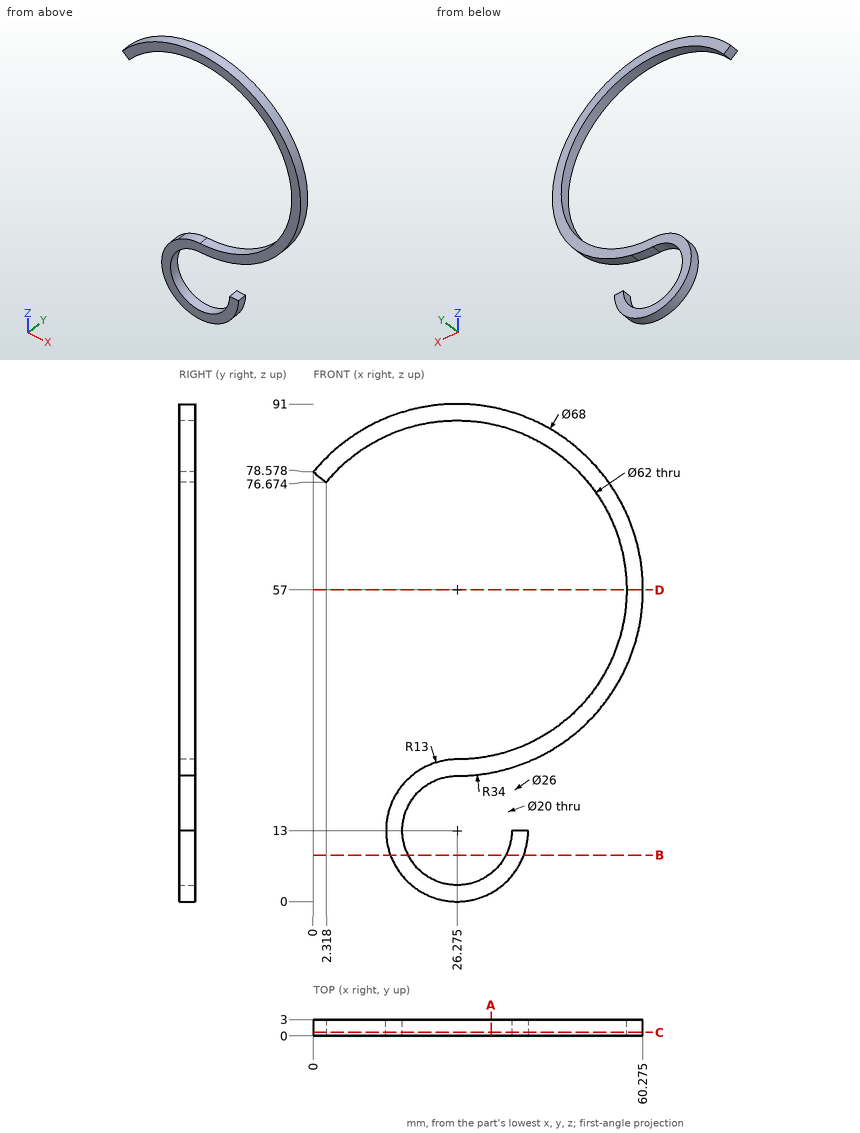
Geometry check sheet. Reference: drawing and pictorial views, mm from the part's lowest x, y, z. Give positions to 0.01 mm unless a question says otherwise; leave off trailing zeros. Write each loop counter-clockwise with the first axis right and the second up, starting at its lowest first coordinate (ties: lowest second). Pieces come first, ordered by that corner, then holes. Notation, with made-up numbers: M -27.5,9 L 3.5,9 A18 cw 3.5,29 Z; hole C 89.25,83.5 d2. An arc over 180 degrees is marked long. Put each result on its own line as item: value. Start each with the question number.
1. Section check D-D (z = 57). Record the cut outline in (x, y) (1 decimal).
2. Section check A-A (x = 32.5). Record the cut outline in (y, z) (1 decimal), and give its area (3 significant figures).
3. Go/stop test with flat-tipped pins: pin 1 Ø1.5 at (x, y) = (37.5, 1.5) entering from +Z; pin 2 Ø6 at (x, z) = (20.5, 19) entering from +Y; pin 3 Ø18 at (x, z) = (26.27, 13) entering from -Y. Record where each tip stops, or that it passes through.
4. Section check C-C (y = 0.65). Record the cut outline in (x, z) (1 decimal), and give its area (3 significant figures).
5. Section check B-B (z = 8.5). Record the cut outline in (x, y) (1 decimal), and give its area (3 significant figures).
6. Scan lines: line 1 along Z through (x, y) = (28.5, 0.65); line 2 along Z through (x, y) = (27, 1.5); line 3 along Z through (x, y) = (15, 2.2) (1 decimal). Record each from-to range of solid material in increasing order. Write a range as [from, to].
Answer list:
1. outline: M 57.3,0 L 60.3,0 L 60.3,3 L 57.3,3 Z
2. outline: M 0,1.6 L 3,1.6 L 3,5.2 L 0,5.2 Z; M 0,23.6 L 3,23.6 L 3,26.6 L 0,26.6 Z; M 0,87.4 L 3,87.4 L 3,90.4 L 0,90.4 Z
2. area: 29.1 mm2
3. pin 1: z = 89.35
3. pin 2: y = 3
3. pin 3: through
4. outline: M 0,78.6 L 2.3,76.7 A31 cw long 26.3,26 A13 ccw long 39.3,13 L 36.3,13 A10 cw long 26.3,23 A34 ccw long Z
4. area: 555 mm2
5. outline: M 14.1,0 L 17.3,0 L 17.3,3 L 14.1,3 Z; M 35.2,0 L 38.5,0 L 38.5,3 L 35.2,3 Z
5. area: 19.6 mm2
6. line 1: [0.19, 3.25], [23.07, 26.08], [87.92, 90.93]
6. line 2: [0.02, 3.03], [23.01, 26.01], [87.99, 90.99]
6. line 3: [6.5, 19.5], [85.9, 89.1]
